Autodesk Inventor part; units mm, degrees
ref_plane "YZ Plane" through (0, 0, 0) normal (1, 0, 0) x (0, 1, 0)
ref_plane "XZ Plane" through (0, 0, 0) normal (0, 1, 0) x (-1, 0, 0)
ref_plane "XY Plane" through (0, 0, 0) normal (0, 0, 1) x (1, 0, 0)
sketch "Sketch1" plane through (0, 0, 0) normal (1, 0, 0) x (0, 1, 0)
  line L0 (0, -20.5) -> (0, 7.5)
  line L1 (-20.7, 0) -> (8.7, 0)
  line L2 (4.5, 3.5) -> (-16.5, 3.5)
  line L3 (-16.5, 3.5) -> (-16.5, -16.5)
  line L4 (-16.5, -16.5) -> (4.5, -16.5)
  line L5 (4.5, -16.5) -> (4.5, 3.5)
  point P0 (0, 0)
  dimension "d0" = 4.5
  dimension "d1" = 20
  dimension "d2" = 21
  dimension "d3" = 3.5
extrude "Extrusion1" add sketch "Sketch1" along normal mid plane 11.5
sketch "Sketch2" plane through (0, 0, 0) normal (0, 0, 1) x (1, 0, 0)
  line L0 (5.75, 4.5) -> (-5.75, 4.5)
  line L1 (-5.75, 4.5) -> (5.75, 4.5)
  line L2 (-5.75, -16.5) -> (5.75, -16.5)
  line L3 (-5.75, -16.5) -> (5.75, -16.5)
  line L4 (-5.75, 4.5) -> (5.75, 4.5)
  line L5 (4.6, 8.8) -> (-4.6, 8.8)
  line L6 (-5.75, -16.5) -> (5.75, -16.5)
  circle A0 centre (0, 6.875) radius 0.925
  line L7 (0, -26.72) -> (0, 14.72)
  line L8 (-5.75, -16.5) -> (-5.75, 4.5)
  line L9 (5.75, 4.5) -> (5.75, -16.5)
  line L10 (-5.75, -6) -> (5.75, -6) construction
  circle A1 centre (0, -18.875) radius 0.925
  line L11 (-4.6, 8.8) -> (-4.6, 4.5)
  line L12 (4.6, 8.8) -> (4.6, 4.5)
  line L13 (-4.6, -16.5) -> (-4.6, -20.8)
  line L14 (-4.6, -20.8) -> (4.6, -20.8)
  line L15 (4.6, -20.8) -> (4.6, -16.5)
  point P0 (0, 0)
  point P1 (0, 7.8)
  dimension "d7" = 1.85
  dimension "d8" = 3.3
  dimension "d12" = 9.2
  dimension "d13" = 4.3
extrude "Extrusion2" add sketch "Sketch2" against normal blind 1 contours L0 L7 A0 L5 L12 | L0 L11 L5 L7 A0 | L15 L14 L7 A1 L2 | L7 A1 L14 L13 L2
fillet "Fillet1" radius 3 4 edges at (4.6, 8.8, -0.5) (-4.6, 8.8, -0.5) (-4.6, -20.8, -0.5) (4.6, -20.8, -0.5)
fillet "Fillet2" radius 0.5 4 edges at (5.75, -16.5, -6.5) (-5.75, -16.5, -6.5) (-5.75, 4.5, -6.5) (5.75, 4.5, -6.5)
sketch "Sketch3" plane through (-5.25, 4.5, 3.5) normal (0, 0, 1) x (1, 0, 0)
  line L0 (11, -0.5) -> (11, -20.5)
  line L1 (5.25, -5.75) -> (5.25, -11.25) construction
  circle A0 centre (5.25, -11.25) radius 3
  line L2 (10.5, 0) -> (0, 0)
  line L3 (-0.5, -20.5) -> (-0.5, -0.5)
  circle A1 centre (5.25, -5.75) radius 5.75
  point P0 (5.25, -4.5)
  dimension "d16" = 6
  dimension "d17" = 5.5
extrude "Extrusion3" add sketch "Sketch3" along normal blind 3.45
sketch "Sketch4" plane through (-5.25, 4.5, 6.95) normal (0, 0, 1) x (1, 0, 0)
  arc A0 (8.1968, -10.6875) -> (2.3032, -10.6875) centre (5.25, -5.75) ccw
  circle A1 centre (5.25, -5.75) radius 1.875
  point P0 (5.25, -4.5)
  dimension "d20" = 3.75
extrude "Extrusion4" add sketch "Sketch4" along normal blind 2.45
properties part number "empty"
Verification items for the finished model (mm, model axes). A direction names the side the tool comes from. Coordinates: 2 decimals unless noted, no trailing zeros. Order: outer loops, then holes, each group sorted by start corner. A loop starts at its lowest first (then second) coordinate and runs counter-clockwise, first axis right, second up. Notation, with made-up numbers: M 22,-23 L 75,-23 A24 ccw 75,1 Z; hole C 16.25,35.25 d6. An arc over 180 degrees is marked long. One line per item, written item: value. Start each with the question number.
Item 1: Sectioned sample at C-C (x = 4). Enter the section's corners in (y, z), then the cut area to 3 significant figures.
Item 2: Sectioned sample at A-A (z = -11.25). Enter the section's corners in (x, y).
Item 3: Access from +Z, -Z, +X, -X, +Y, -Y to the whole of each face (thin tool, end or side, straight path). Record for faces 5 (the flat face through (0, -12, 3.5)), 6 (the flat face through (4.4, 3.1, 3.5)), 7 (the flat face through (-0.1, 5.7, 0)), 8 (the flat face through (-0.1, -17.7, -1)), 9 (the flat face through (4.6, -17.2, -0.5)).
Item 4: Scan lines: probe 1 along Y at (x, z) = (0, -0.5); probe 2 along Z at (x, y) = (2.5, -10.25); probe 3 along Z at (x, y) = (1, 1.75). Record each from-to range of solid material in increasing order.
Item 5: Mould release check, pull along Y, two halves, no side actions. Record for faces 1 (the cylindrical face through (-0.24, -3.11, 8.16)), 2 (the cylindrical face through (-3.74, 7.9, -0.51)), 3 (the cylindrical face through (0.882, 7.153, -0.493)), 4 (the flat face through (-4.6, -17.1, -0.5)): released by +Y, released by -Y, zero draft, split by the parting line, or undercut.
Item 6: Gauge pin test, flat ends, axial feed: pin 1 (2 mm diameter, centred on x = 2, y = -19.5, fed in from +Z); pin 2 (3 mm diameter, centred on x = 4, y = -14.5, fed in from +Z); pin 3 (0.5 mm diameter, centred on y = -17.5, z = -0.5, fed in from -X). Record the tip position at first contact, or that the pin passes through.
Item 7: Sectioned sample at D-D (y = 0). Enter the section's corners in (x, z).
Item 8: Sectioned sample at B-B (y = -6.75). Enter the section's corners in (x, z).
Conclusion:
1. outline: M -19.6,-1 L -16.5,-1 L -16.5,-16.5 L 4.5,-16.5 L 4.5,-1 L 7.6,-1 L 7.6,0 L 4.5,0 L 4.5,3.5 L 2.88,3.5 L 2.88,6.95 L -5.38,6.95 L -5.38,3.5 L -16.5,3.5 L -16.5,0 L -19.6,0 Z
1. area: 455 mm^2
2. outline: M -5.75,-16 A0.5 ccw -5.25,-16.5 L 5.25,-16.5 A0.5 ccw 5.75,-16 L 5.75,4 A0.5 ccw 5.25,4.5 L -5.25,4.5 A0.5 ccw -5.75,4 Z
3. face 5: +Z, -Y
3. face 6: +Z, +X, +Y
3. face 7: +Z, +X, -X, +Y
3. face 8: -Z, +X, -X, -Y
3. face 9: +Z, -Z, +X, -Y
4. probe 1: y = -20.8 to -19.8, -17.95 to 5.95, 7.8 to 8.8
4. probe 2: z = -16.5 to 3.5
4. probe 3: z = -16.5 to 6.95
5. face 1: split by the parting line
5. face 2: released by +Y
5. face 3: undercut
5. face 4: zero draft
6. pin 1: stops at z = 0
6. pin 2: stops at z = 3.5
6. pin 3: stops at x = -4.6
7. outline: M -5.75,-16.5 L 5.75,-16.5 L 5.75,3.5 L 5.61,3.5 L 5.61,6.95 L 1.4,6.95 L 1.4,9.4 L -1.4,9.4 L -1.4,6.95 L -5.61,6.95 L -5.61,3.5 L -5.75,3.5 Z
8. outline: M -5.75,-16.5 L 5.75,-16.5 L 5.75,3.5 L 3,3.5 L 3,6.95 L -3,6.95 L -3,3.5 L -5.75,3.5 Z
